from build123d import *


with BuildPart() as f5:
    # F0 (on Right) → F5 (revolve)
    with BuildSketch(Plane.YZ):
        with BuildLine():
            Line((-52.6758568757, 24.765), (-59.055, 21.082))
            Line((-59.055, 21.082), (-20.955, 21.082))
            Line((-20.955, 21.082), (-20.955, 15.875))
            Line((-20.955, 15.875), (0, 15.875))
            ThreePointArc((0, 15.875), (11.2253201513, 11.2253201513), (15.875, 0))
            Line((15.875, 0), (24.765, 0))
            ThreePointArc((24.765, 0), (17.5114994361, 17.5114994361), (0, 24.765))
            Line((0, 24.765), (-52.6758568757, 24.765))
        make_face()
        with BuildLine():
            Line((-20.955, 21.082), (-59.055, 21.082))
            Line((-59.055, 21.082), (-59.055, 0))
            Line((-59.055, 0), (0, 0))
            Line((0, 0), (10.5189766587, 0))
            Line((10.5189766587, 0), (15.875, 0))
            ThreePointArc((15.875, 0), (11.2253201513, 11.2253201513), (0, 15.875))
            Line((0, 15.875), (-20.955, 15.875))
            Line((-20.955, 15.875), (-20.955, 21.082))
        make_face()
    revolve(axis=Axis((0, -21.59, 0), (0, 1, 0)))

    # F1 (on Right) → F6 (revolve)
    with BuildSketch(Plane.YZ):
        with BuildLine():
            Line((-24.765, -52.6758568757), (-21.082, -59.055))
            Line((-21.082, -59.055), (-21.082, -20.955))
            Line((-21.082, -20.955), (-15.875, -20.955))
            Line((-15.875, -20.955), (-15.875, 0))
            ThreePointArc((-15.875, 0), (-11.2253201513, 11.2253201513), (0, 15.875))
            Line((0, 15.875), (0, 24.765))
            ThreePointArc((0, 24.765), (-17.5114994361, 17.5114994361), (-24.765, 0))
            Line((-24.765, 0), (-24.765, -52.6758568757))
        make_face()
        with BuildLine():
            Line((-21.082, -20.955), (-21.082, -59.055))
            Line((-21.082, -59.055), (0, -59.055))
            Line((0, -59.055), (0, 0))
            Line((0, 0), (0, 15.875))
            ThreePointArc((0, 15.875), (-11.2253201513, 11.2253201513), (-15.875, 0))
            Line((-15.875, 0), (-15.875, -20.955))
            Line((-15.875, -20.955), (-21.082, -20.955))
        make_face()
    revolve(axis=Axis((0, 0, -21.59), (0, 0, 1)))

    # F2 (on Right) → F7 (revolve)
    with BuildSketch(Plane.YZ):
        with BuildLine():
            Line((52.6758568757, -24.765), (59.055, -21.082))
            Line((59.055, -21.082), (20.955, -21.082))
            Line((20.955, -21.082), (20.955, -15.875))
            Line((20.955, -15.875), (0, -15.875))
            ThreePointArc((0, -15.875), (-11.2253201513, -11.2253201513), (-15.875, 0))
            Line((-15.875, 0), (-24.765, 0))
            ThreePointArc((-24.765, 0), (-17.5114994361, -17.5114994361), (0, -24.765))
            Line((0, -24.765), (52.6758568757, -24.765))
        make_face()
        with BuildLine():
            Line((20.955, -21.082), (59.055, -21.082))
            Line((59.055, -21.082), (59.055, 0))
            Line((59.055, 0), (10.5189766587, 0))
            Line((10.5189766587, 0), (0, 0))
            Line((0, 0), (-15.875, 0))
            ThreePointArc((-15.875, 0), (-11.2253201513, -11.2253201513), (0, -15.875))
            Line((0, -15.875), (20.955, -15.875))
            Line((20.955, -15.875), (20.955, -21.082))
        make_face()
    revolve(axis=Axis((0, 21.59, 0), (0, -1, 0)))

    # F3 (on Right) → F8 (revolve)
    with BuildSketch(Plane.YZ):
        with BuildLine():
            Line((24.765, 52.6758568757), (21.082, 59.055))
            Line((21.082, 59.055), (21.082, 20.955))
            Line((21.082, 20.955), (15.875, 20.955))
            Line((15.875, 20.955), (15.875, 0))
            ThreePointArc((15.875, 0), (11.2253201513, -11.2253201513), (0, -15.875))
            Line((0, -15.875), (0, -24.765))
            ThreePointArc((0, -24.765), (17.5114994361, -17.5114994361), (24.765, 0))
            Line((24.765, 0), (24.765, 52.6758568757))
        make_face()
        with BuildLine():
            Line((21.082, 20.955), (21.082, 59.055))
            Line((21.082, 59.055), (0, 59.055))
            Line((0, 59.055), (0, 9.2996467855))
            Line((0, 9.2996467855), (0, 0))
            Line((0, 0), (0, -15.875))
            ThreePointArc((0, -15.875), (11.2253201513, -11.2253201513), (15.875, 0))
            Line((15.875, 0), (15.875, 20.955))
            Line((15.875, 20.955), (21.082, 20.955))
        make_face()
    revolve(axis=Axis((0, 0, 21.59), (0, 0, -1)))

    # F4 (on Top) → F9 (revolve)
    with BuildSketch(Plane.XY):
        with BuildLine():
            Line((-52.6758568757, 24.765), (-59.055, 21.082))
            Line((-59.055, 21.082), (-20.955, 21.082))
            Line((-20.955, 21.082), (-20.955, 15.875))
            Line((-20.955, 15.875), (0, 15.875))
            ThreePointArc((0, 15.875), (11.2253201513, 11.2253201513), (15.875, 0))
            Line((15.875, 0), (24.765, 0))
            ThreePointArc((24.765, 0), (17.5114994361, 17.5114994361), (0, 24.765))
            Line((0, 24.765), (-52.6758568757, 24.765))
        make_face()
        with BuildLine():
            Line((-20.955, 21.082), (-59.055, 21.082))
            Line((-59.055, 21.082), (-59.055, 0))
            Line((-59.055, 0), (-12.5608257832, 0))
            Line((-12.5608257832, 0), (0, 0))
            Line((0, 0), (15.875, 0))
            ThreePointArc((15.875, 0), (11.2253201513, 11.2253201513), (0, 15.875))
            Line((0, 15.875), (-20.955, 15.875))
            Line((-20.955, 15.875), (-20.955, 21.082))
        make_face()
    revolve(axis=Axis((-21.59, 0, 0), (1, 0, 0)))

    # F0 (on Right) → F10 (revolve, cut)
    with BuildSketch(Plane.YZ):
        with BuildLine():
            Line((-20.955, 21.082), (-59.055, 21.082))
            Line((-59.055, 21.082), (-59.055, 0))
            Line((-59.055, 0), (0, 0))
            Line((0, 0), (10.5189766587, 0))
            Line((10.5189766587, 0), (15.875, 0))
            ThreePointArc((15.875, 0), (11.2253201513, 11.2253201513), (0, 15.875))
            Line((0, 15.875), (-20.955, 15.875))
            Line((-20.955, 15.875), (-20.955, 21.082))
        make_face()
    revolve(axis=Axis((0, -21.59, 0), (0, 1, 0)), mode=Mode.SUBTRACT)

    # F1 (on Right) → F11 (revolve, cut)
    with BuildSketch(Plane.YZ):
        with BuildLine():
            Line((-21.082, -20.955), (-21.082, -59.055))
            Line((-21.082, -59.055), (0, -59.055))
            Line((0, -59.055), (0, 0))
            Line((0, 0), (0, 15.875))
            ThreePointArc((0, 15.875), (-11.2253201513, 11.2253201513), (-15.875, 0))
            Line((-15.875, 0), (-15.875, -20.955))
            Line((-15.875, -20.955), (-21.082, -20.955))
        make_face()
    revolve(axis=Axis((0, 0, -21.59), (0, 0, 1)), mode=Mode.SUBTRACT)

    # F2 (on Right) → F12 (revolve, cut)
    with BuildSketch(Plane.YZ):
        with BuildLine():
            Line((20.955, -21.082), (59.055, -21.082))
            Line((59.055, -21.082), (59.055, 0))
            Line((59.055, 0), (10.5189766587, 0))
            Line((10.5189766587, 0), (0, 0))
            Line((0, 0), (-15.875, 0))
            ThreePointArc((-15.875, 0), (-11.2253201513, -11.2253201513), (0, -15.875))
            Line((0, -15.875), (20.955, -15.875))
            Line((20.955, -15.875), (20.955, -21.082))
        make_face()
    revolve(axis=Axis((0, 21.59, 0), (0, -1, 0)), mode=Mode.SUBTRACT)

    # F3 (on Right) → F13 (revolve, cut)
    with BuildSketch(Plane.YZ):
        with BuildLine():
            Line((21.082, 20.955), (21.082, 59.055))
            Line((21.082, 59.055), (0, 59.055))
            Line((0, 59.055), (0, 9.2996467855))
            Line((0, 9.2996467855), (0, 0))
            Line((0, 0), (0, -15.875))
            ThreePointArc((0, -15.875), (11.2253201513, -11.2253201513), (15.875, 0))
            Line((15.875, 0), (15.875, 20.955))
            Line((15.875, 20.955), (21.082, 20.955))
        make_face()
    revolve(axis=Axis((0, 0, 21.59), (0, 0, -1)), mode=Mode.SUBTRACT)

    # F4 (on Top) → F14 (revolve, cut)
    with BuildSketch(Plane.XY):
        with BuildLine():
            Line((-20.955, 21.082), (-59.055, 21.082))
            Line((-59.055, 21.082), (-59.055, 0))
            Line((-59.055, 0), (-12.5608257832, 0))
            Line((-12.5608257832, 0), (0, 0))
            Line((0, 0), (15.875, 0))
            ThreePointArc((15.875, 0), (11.2253201513, 11.2253201513), (0, 15.875))
            Line((0, 15.875), (-20.955, 15.875))
            Line((-20.955, 15.875), (-20.955, 21.082))
        make_face()
    revolve(axis=Axis((-21.59, 0, 0), (1, 0, 0)), mode=Mode.SUBTRACT)


solid = f5.part
The listing builds one solid part. Answer for the finished solid, in the listing's coordinates (mm). A direction names the side the tool comes from. Coordinates: 2 decimals unless noted, no trailing zeros. Loops run counter-clockwise (first coordinate to the right, second up) from the corner with the lowest first, then second, coordinate; pieces in that order, holes last. Notation, with made-up numbers: (15.25, 11.25) -> (26.25, 11.25) arc R19 ccw to (26.25, 48.25) -> close; hole circle Ø7 at (7.5, 1). An arc over 180 degrees is marked (long way). Answer in a Markdown table with one row per item. Add a question column.
1. Determine the mould class of faces 4 (the cylindrical face through (24.554, 32.56, 3.224)), 5 (the conical face through (-58.745, -4.609, -20.755)), 6 (the flat face through (-9, -20.955, -14)), 7 (the cylindrical face through (-40.27, 20.11, 6.33)) for opening direction X: +X half, -X half, draft (parallel to the pull), parting line (faces both ways), or undercut.
2. The part is cut by section B-B, the plane z = -38. Write down the section's boundary in (x, y) (3 decimals).
3. For faces 1 (the flat face through (-20.955, -9, -14)), 2 (the cylindrical face through (6.33, -20.11, -40.27)), 3 (the flat face through (-9, -14, 20.955)), determine the directions among +Z, -Z, +X, -X, +Y, -Y from which every point of the face is accessible in a straight line to the end or side of a thin tool.
4. Flat-ended cylindrical pins translate along their axes: P1, Ø12, axis at y = -25, z = 13, coming from the +X side; P2, Ø3, axis at x = -9.5, z = -11.5, coming from the -Y side (3 decimals); P3, Ø5, axis at x = -43.5, z = 16.5, coming from the +Y side. Find the tip coordinate at first contact, or state that the pin passes through.
5. The part is cut by section A-A, the plane x = 0. Count the separate pieces of the cut face and the enclosed holes in it, then the cut area to 3 significant figures.
6. Consider line 1 (X direction, y = 49, z = 0) (3 decimals); line 2 (Y direction, x = -16, z = -0.5) (3 decimals). Determine where each line is inside the solid, lowest interval first. Write a range as [from, to].
Answer below:
| question | item | result |
|---|---|---|
| 1 | face 4 | parting line |
| 1 | face 5 | -X half |
| 1 | face 6 | undercut |
| 1 | face 7 | draft |
| 2 | outline | circle Ø49.53 at (0, 0); hole circle Ø42.164 at (0, 0) |
| 3 | face 1 | -X |
| 3 | face 2 | -Z |
| 3 | face 3 | +Z |
| 4 | P1 | x = 23.76 |
| 4 | P2 | y = -20.955 |
| 4 | P3 | y = 20.43 |
| 5 | separate pieces | 8 |
| 5 | enclosed holes | 0 |
| 5 | area | 1,070 mm2 |
| 6 | line 1 | [-24.765, -21.082], [21.082, 24.765] |
| 6 | line 2 | [-20.955, -15.867], [15.867, 20.955] |
